Part model, mm, in its own coordinate system. Face numbers are marked on the shaded views. Round coordinates to 2 decimals unless told otherwise and drop trailing zeros. Write each loop counter-clockwise with the first axis right and the second up, starting at its lowest first coordinate (ties: lowest second). Pieces come first, ordered by that corner, then holes. Notation, with made-up numbers: (-13.5, 86.5) -> (-4.5, 86.5) arc R20 cw to (-4.5, 108.5) -> close; hole circle Ø6 at (-17.75, 77.25). An arc over 180 degrees is marked (long way). Use CSV: the item, a comma, the result in double quotes. Start each with the question number.
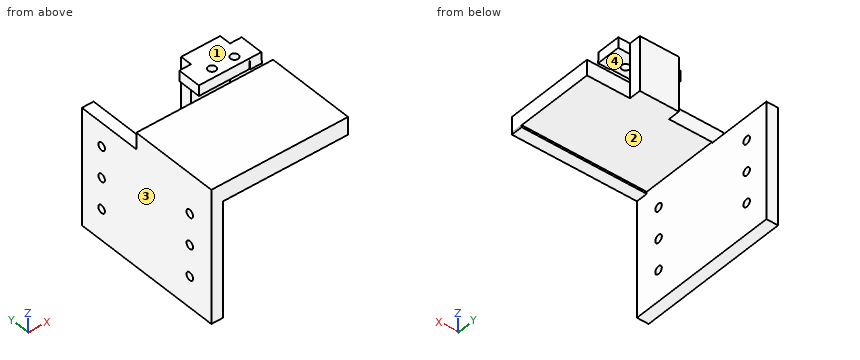
```python
from build123d import *

# Parameters (mm, degrees)
ESQUISSE1_R             = 1
BOSS_EXTRU_1_DEPTH      = 3
ESQUISSE2_W             = 32.050081832
ESQUISSE2_H             = 3
BOSS_EXTRU_2_DEPTH      = 4
ESQUISSE3_W             = 32.050081832
ESQUISSE3_H             = 4
BOSS_EXTRU_3_DEPTH      = 20
BOSS_EXTRU_4_DEPTH      = 10
BOSS_EXTRU_4_DEPTH_BACK = 4
ESQUISSE5_W             = 10
ESQUISSE5_H             = 2.701469748
BOSS_EXTRU_5_DEPTH      = 6
BOSS_EXTRU_6_DEPTH      = 3
ESQUISSE7_W             = 2.701469748
ESQUISSE7_H             = 6
BOSS_EXTRU_7_DEPTH      = 3
ESQUISSE8_R             = 1
ENL_V_MAT_EXTRU_1_DEPTH = 5
ESQUISSE9_W             = 32.395093649
ESQUISSE9_H             = 3
ENL_V_MAT_EXTRU_2_DEPTH = 24
ESQUISSE10_W            = 4.230170434
ESQUISSE10_H            = 23
BOSS_EXTRU_8_DEPTH      = 3
ESQUISSE11_W            = 3
ESQUISSE11_H            = 39.66165995
BOSS_EXTRU_9_DEPTH      = 30
ESQUISSE12_R            = 1
ENL_V_MAT_EXTRU_3_DEPTH = 30


with BuildPart() as part:
    # Esquisse1 → Boss.-Extru.1 (new body)
    with BuildSketch(Plane(origin=(0, 0, 0), x_dir=(1, 0, 0), z_dir=(0, 1, 0))):
        Polygon((-38.959245403, 34.630440358), (-6.759245403, 34.630440358), (-6.909163571, 10.109841365), (-38.959245403, 10.109841365), align=None)
        with Locations(Location((-36.509163571, 15.109841365, 0), (0, 0, 270))):
            Circle(ESQUISSE1_R, mode=Mode.SUBTRACT)
        with Locations(Location((-9.509163571, 15.109841365, 0), (0, 0, 270))):
            Circle(ESQUISSE1_R, mode=Mode.SUBTRACT)
        with Locations(Location((-36.509163571, 23.109841365, 0), (0, 0, 270))):
            Circle(ESQUISSE1_R, mode=Mode.SUBTRACT)
        with Locations(Location((-9.509163571, 23.109841365, 0), (0, 0, 270))):
            Circle(ESQUISSE1_R, mode=Mode.SUBTRACT)
        with Locations(Location((-36.509163571, 31.109841365, 0), (0, 0, 270))):
            Circle(ESQUISSE1_R, mode=Mode.SUBTRACT)
        with Locations(Location((-9.509163571, 31.109841365, 0), (0, 0, 270))):
            Circle(ESQUISSE1_R, mode=Mode.SUBTRACT)
    extrude(amount=BOSS_EXTRU_1_DEPTH)

    # Esquisse2 → Boss.-Extru.2 (add)
    with BuildSketch(Plane.XY.offset(-10.109841365)):
        with Locations((-22.934204487, 1.5)):
            Rectangle(ESQUISSE2_W, ESQUISSE2_H)
    extrude(amount=BOSS_EXTRU_2_DEPTH)

    # Esquisse3 → Boss.-Extru.3 (add)
    with BuildSketch(Plane(origin=(0, 3, 0), x_dir=(1, 0, 0), z_dir=(0, 1, 0))):
        with Locations((-22.934204487, 8.109841365)):
            Rectangle(ESQUISSE3_W, ESQUISSE3_H)
    extrude(amount=BOSS_EXTRU_3_DEPTH)

    # Esquisse4 → Boss.-Extru.4 (add, two sides: drawn at the far end of the back side and taken through both)
    with BuildSketch(Plane.XY.offset(-6.109841365).offset(-BOSS_EXTRU_4_DEPTH_BACK)):
        Polygon((-22.934204487, 23), (-17.934204487, 23), (-17.934204487, 26), (-27.934204487, 26), (-27.934204487, 23), align=None)
    extrude(amount=BOSS_EXTRU_4_DEPTH + BOSS_EXTRU_4_DEPTH_BACK)

    # Esquisse5 → Boss.-Extru.5 (add)
    with BuildSketch(Plane.XZ.offset(-23)):
        with Locations((-22.934204487, 2.539423761)):
            Rectangle(ESQUISSE5_W, ESQUISSE5_H)
    extrude(amount=BOSS_EXTRU_5_DEPTH)

    # Esquisse6 → Boss.-Extru.6 (add)
    with BuildSketch(Plane(origin=(-17.934204487, 0, 0), x_dir=(0, 0, -1), z_dir=(1, 0, 0))):
        Polygon((-1.188688887, 23), (-3.890158635, 23), (-3.890158635, 17), (-1.188688887, 16.813684491), align=None)
    extrude(amount=BOSS_EXTRU_6_DEPTH)

    # Esquisse7 → Boss.-Extru.7 (add)
    with BuildSketch(Plane.ZY.offset(27.934204487)):
        with Locations((2.539423761, 20)):
            Rectangle(ESQUISSE7_W, ESQUISSE7_H)
    extrude(amount=BOSS_EXTRU_7_DEPTH)

    # Esquisse8 → Enlèv. mat.-Extru.1 (cut)
    with BuildSketch(Plane.XY.offset(3.890158635)):
        with Locations((-25.616934949, 19.323429725)):
            Circle(ESQUISSE8_R)
        with Locations((-19.884204487, 19.323429725)):
            Circle(ESQUISSE8_R)
    extrude(amount=-ENL_V_MAT_EXTRU_1_DEPTH, mode=Mode.SUBTRACT)

    # Esquisse9 → Enlèv. mat.-Extru.2 (cut)
    with BuildSketch(Plane(origin=(0, 0, -34.630440358), x_dir=(-1, 0, 0), z_dir=(0, 0, -1))):
        with Locations((22.956792228, 1.5)):
            Rectangle(ESQUISSE9_W, ESQUISSE9_H)
    extrude(amount=-ENL_V_MAT_EXTRU_2_DEPTH, mode=Mode.SUBTRACT)

    # Esquisse10 → Boss.-Extru.8 (add)
    with BuildSketch(Plane.ZY.offset(38.959245403)):
        with Locations((-8.224926582, 11.5)):
            Rectangle(ESQUISSE10_W, ESQUISSE10_H)
    extrude(amount=BOSS_EXTRU_8_DEPTH)

    # Esquisse11 → Boss.-Extru.9 (add)
    with BuildSketch(Plane(origin=(0, 0, -10.340011799), x_dir=(-1, 0, 0), z_dir=(0, 0, -1))):
        with Locations((40.459245403, 19.830829975)):
            Rectangle(ESQUISSE11_W, ESQUISSE11_H)
    extrude(amount=BOSS_EXTRU_9_DEPTH)

    # Esquisse12 → Enlèv. mat.-Extru.3 (cut)
    with BuildSketch(Plane(origin=(-41.959245403, -0.142686019, -42.326053617), x_dir=(0, -1, 0), z_dir=(-1, 0, 0))):
        with Locations(Location((-33.753075005, 25.951540398, 0), (0, 0, 90))):
            Circle(ESQUISSE12_R)
        with Locations(Location((-33.753075005, 17.951540398, 0), (0, 0, 90))):
            Circle(ESQUISSE12_R)
        with Locations(Location((-6.753075005, 25.951540398, 0), (0, 0, 90))):
            Circle(ESQUISSE12_R)
        with Locations(Location((-6.753075005, 17.951540398, 0), (0, 0, 90))):
            Circle(ESQUISSE12_R)
        with Locations(Location((-6.753075005, 9.951540398, 0), (0, 0, 90))):
            Circle(ESQUISSE12_R)
        with Locations(Location((-33.753075005, 9.951540398, 0), (0, 0, 90))):
            Circle(ESQUISSE12_R)
    extrude(amount=-ENL_V_MAT_EXTRU_3_DEPTH, mode=Mode.SUBTRACT)


solid = part.part
```
1. Flat gauge pins, fed straight in: pin 1 (5 mm diameter, centred on x = -24.5, y = 10, fed in from -Z); pin 2 (3 mm diameter, centred on x = -17, z = 2.5, fed in from +Y); pin 3 (12 mm diameter, centred on y = 31.5, z = -35.5, fed in from +X). Where does each tip first touch, or does it go through?
2. Band-saw the part on A-A (x = -29). List the corners of the cut face in (y, z), then the cut area to 3 significant figures.
3. Band-saw the part on B-B (z = -24). List the corners of the cut face in (x, y).
4. Band-saw the part on C-C (x = -13.5). List the corners of the cut face in (y, z).
5. Drill centre lines: line 1 along X through (y, z) = (20, -23); line 2 along Z through (x, y) = (-15.5, 13); line 3 along Z through (x, y) = (-39, 28). Where is each one in solid material? Low to high. Write a range as [from, to].
6. Band-saw the part on D-D (y = 13). List the corners of the cut face in (x, z).
7. Pull direction Z, two halves, no side cores. Call the marked faces 1, 2, 3 and 4: released by +Z, released by -Z, zero draft, split by the parting line, or undercut.
Answers below:
1,pin 1,"stops at z = -10.11"
1,pin 2,"stops at y = 26"
1,pin 3,"stops at x = -38.96"
2,outline,"(0, -10.63) -> (3, -10.63) -> (3, -10.11) -> (23, -10.11) -> (23, -6.11) -> (0, -6.11) -> close; (17, 1.19) -> (23, 1.19) -> (23, 3.89) -> (17, 3.89) -> close"
2,area,"110 mm^2"
3,outline,"(-41.96, 0) -> (-38.96, 0) -> (-38.96, 5.68) -> (-41.96, 5.68) -> close; (-41.96, 7.54) -> (-38.96, 7.54) -> (-38.96, 32.68) -> (-41.96, 32.68) -> close; (-41.96, 34.54) -> (-38.96, 34.54) -> (-38.96, 39.66) -> (-41.96, 39.66) -> close"
4,outline,"(0, -10.63) -> (3, -10.63) -> (3, -10.11) -> (23, -10.11) -> (23, -6.11) -> (0, -6.11) -> close"
5,line 1,"x = [-41.96, -38.96]"
5,line 2,"z = [-10.11, -6.11]"
5,line 3,"z = [-40.34, -10.34]"
6,outline,"(-41.96, -40.34) -> (-38.96, -40.34) -> (-38.96, -10.11) -> (-6.91, -10.11) -> (-6.91, -6.11) -> (-41.96, -6.11) -> close"
7,face 1,"released by +Z"
7,face 2,"released by -Z"
7,face 3,"zero draft"
7,face 4,"undercut"
